Study the drawing (mm; zero at the part's minimum x, y, z) and answer. A direction names the side the tool comes from. Give positions to 0.01 mm unless a question says otherwise; leave off trailing zeros. Order: outer loops, then holes, each group sorted by start corner. A loop starts at its lowest first (then second) coordinate and runs counter-clockwise, first axis right, second up.
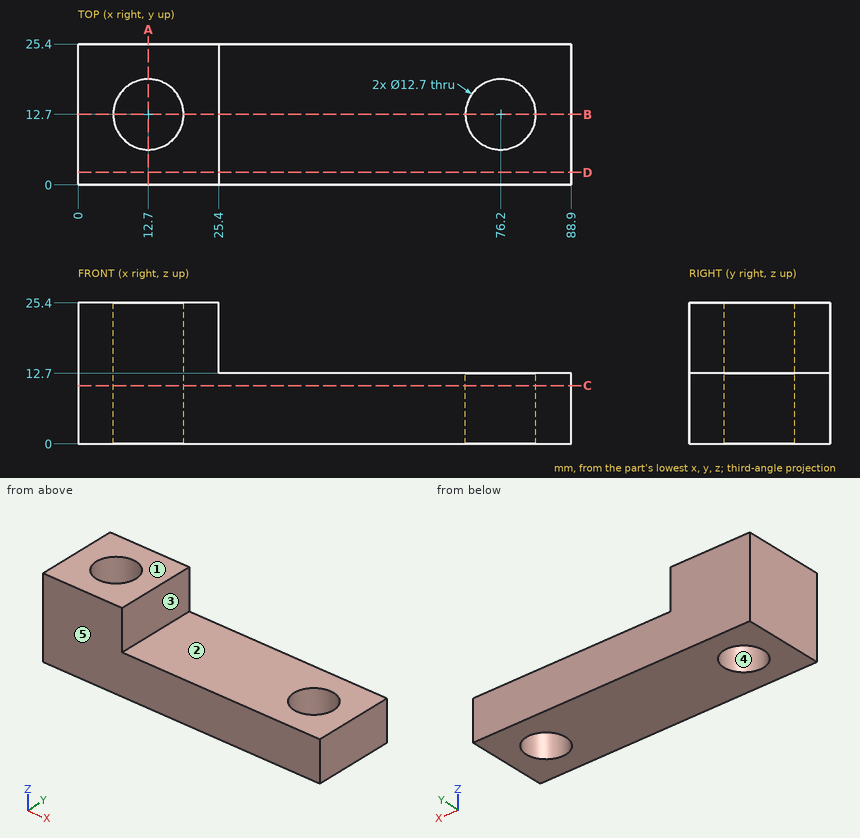
1) Find section A-A (x = 12.7). Write down the section's boundary in (y, z).
Geometry says:
outline: (0, 0) - (6.35, 0) - (6.35, 25.4) - (0, 25.4) - close; (19.05, 0) - (25.4, 0) - (25.4, 25.4) - (19.05, 25.4) - close
2) Straight lines are drawn through the part: probe 1 along Y at (x, z) = (12.7, 6.25); probe 2 along X at (y, z) = (8.25, 5.25); probe 3 along Z at (x, y) = (71, 19). For each, find the intervals that lie inside material, in ascending order.
Geometry says:
probe 1: y = 0 to 6.35, 19.05 to 25.4
probe 2: x = 0 to 8.17, 17.23 to 71.67, 80.73 to 88.9
probe 3: z = 0 to 12.7
3) A tool of negligible diameter and unlimited length cuts with its end or side. For the marked faces 1 and 2, from which of +Z, -Z, +X, -X, +Y, -Y can it reach the whole face along a straight path? Write none if from no direction.
Geometry says:
face 1: +Z, +X, -X, +Y, -Y
face 2: +Z, +X, +Y, -Y
4) Find section B-B (y = 12.7). Write down the section's boundary in (x, z), then the cut area to 3 significant figures.
Geometry says:
outline: (0, 0) - (6.35, 0) - (6.35, 25.4) - (0, 25.4) - close; (19.05, 0) - (69.85, 0) - (69.85, 12.7) - (25.4, 12.7) - (25.4, 25.4) - (19.05, 25.4) - close; (82.55, 0) - (88.9, 0) - (88.9, 12.7) - (82.55, 12.7) - close
area: 968 mm2
5) Find section C-C (z = 10.5). Write down the section's boundary in (x, y), then the cut area to 3 significant figures.
Geometry says:
outline: (0, 0) - (88.9, 0) - (88.9, 25.4) - (0, 25.4) - close; hole circle Ø12.7 at (12.7, 12.7); hole circle Ø12.7 at (76.2, 12.7)
area: 2,000 mm2
6) Given P1, Ø10, axis at x = 48, y = 11.5, coming from the +Z side; P2, Ø10, axis at y = 12, z = 22, coming from the +X side, each flat-ended and moving along its own axis, determine where each tip first touches the part or whether it passes through.
Geometry says:
P1: stops at z = 12.7
P2: stops at x = 25.4
7) Find section D-D (y = 2.25). Write down the section's boundary in (x, z).
Geometry says:
outline: (0, 0) - (88.9, 0) - (88.9, 12.7) - (25.4, 12.7) - (25.4, 25.4) - (0, 25.4) - close
8) For a pull along Y with two mould halves and no side action, classify the marked faces 3, 4 and 5 as +Y half, -Y half, draft (parallel to the pull), parting line (faces both ways), or undercut.
Geometry says:
face 3: draft
face 4: undercut
face 5: -Y half
